The model under review builds one solid part; all positions refer to its coordinate system, in mm. Face numbers are marked on the shaded views. A direction names the side the tool comes from. Coordinates: 2 decimals unless noted, no trailing zeros. Loops run counter-clockwise (first coordinate to the right, second up) from the corner with the lowest first, then second, coordinate; pieces in that order, holes last. Notation, with made-up numbers: (4.25, 63.25) - (19.25, 63.25) arc R20 ccw to (19.25, 99.25) - close; hole circle Ø6 at (29.25, 47). An arc over 180 degrees is marked (long way). Answer in a Markdown table with one row per item. Add a question column.
(1) We need section C-C on y = 2. Write out the cut boundary in (x, z).
(2) We need section D-D on x = 0. Write out the cut boundary in (y, z).
(3) We need section B-B on z = 16. Write out the cut boundary in (x, y), plus the area to 3 significant figures.
(4) For line 1 along X through (y, z) = (0, 48); line 2 along Z through (x, y) = (-6, -19); line 3 along Y through (x, z) = (9, 0.7), list the stretches that pass through material, from the lowest coordinate up.
(5) We need section A-A on x = -15. Write out the cut boundary in (y, z) (1 decimal).
(6) For P1, Ø3, axis at x = 13.5, z = 51, coming from the -Y side; P2, Ø0.5, axis at x = 22.5, z = 76.5, coming from the -Y side; P3, Ø1, axis at y = -7, z = 16.5, coming from the +X side; P4, Ø6, axis at x = 15.5, y = -12, coming from the +Z side, all flat-tipped, find the tip position at first contact; note any pin that passes through.
(7) Machinability: for the marked faces 1 and 2, which of the approach directions +Z, -Z, +X, -X, +Y, -Y give a long, thin tool a straight path to every point of the face, cutting with its end or side? Answer none if there is none.
from build123d import *

# Parameters (mm, degrees)
F0_R     = 24
F1_DEPTH = 3
F2_R     = 24
F2_R_2   = 22.5
F3_DEPTH = 80
F4_W     = 13
F4_H     = 13
F4_R     = 4.75
F5_DEPTH = 3.001
F6_W     = 3.55
F6_H     = 10
F7_DEPTH = 25


with BuildPart() as f1:
    # F0 (on Top) → F1 (new body)
    with BuildSketch(Plane.XY):
        Circle(F0_R)
    extrude(amount=F1_DEPTH)

    # F2 (on face) → F3 (join)
    with BuildSketch(Plane.XY.offset(3)):
        Circle(F2_R)
        Circle(F2_R_2, mode=Mode.SUBTRACT)
    extrude(amount=F3_DEPTH)

    # F4 (on face) → F5 (cut, through all)
    with BuildSketch(Plane.XY.offset(3)):
        with Locations((-9.5, 0)):
            Rectangle(F4_W, F4_H)
        with Locations((9, 0)):
            Circle(F4_R)
    extrude(amount=-F5_DEPTH, mode=Mode.SUBTRACT)

    # F6 (on Right) → F7 (cut)
    with BuildSketch(Plane.YZ):
        with Locations((1.775, 78)):
            Rectangle(F6_W, F6_H)
    extrude(amount=F7_DEPTH, mode=Mode.SUBTRACT)


solid = f1.part
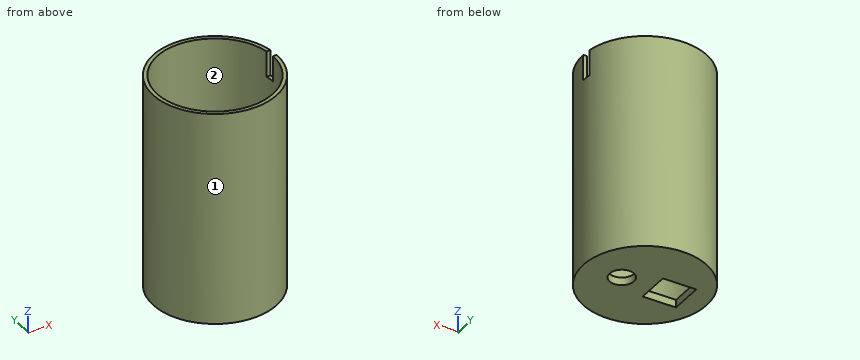
Outcome:
| question | item | result |
|---|---|---|
| 1 | outline | (-23.92, 0) - (-16, 0) - (-16, 3) - (-22.41, 3) - (-22.41, 83) - (-23.92, 83) - close; (-3, 0) - (4.69, 0) - (4.69, 3) - (-3, 3) - close; (13.31, 0) - (23.92, 0) - (23.92, 73) - (22.41, 73) - (22.41, 3) - (13.31, 3) - close |
| 2 | outline | (-24, 0) - (24, 0) - (24, 83) - (22.5, 83) - (22.5, 3) - (-22.5, 3) - (-22.5, 83) - (-24, 83) - close |
| 3 | outline | circle Ø48 at (0, 0); hole circle Ø45 at (0, 0) |
| 3 | area | 219 mm² |
| 4 | line 1 | -24 to -22.5, 22.5 to 24 |
| 4 | line 2 | 0 to 3 |
| 4 | line 3 | -22.25 to -4.75, 4.75 to 22.25 |
| 5 | outline | (-18.7, 0) - (-6.5, 0) - (-6.5, 3) - (-16.8, 3) - (-16.8, 83) - (-18.7, 83) - close; (6.5, 0) - (18.7, 0) - (18.7, 83) - (16.8, 83) - (16.8, 3) - (6.5, 3) - close |
| 6 | P1 | y = -20.78 |
| 6 | P2 | y = -9 |
| 6 | P3 | x = 23.1 |
| 6 | P4 | z = 83 |
| 7 | face 1 | +Z, -Z |
| 7 | face 2 | +Z |
